Autodesk Inventor part; units mm, degrees
ref_plane "YZ Plane" through (0, 0, 0) normal (1, 0, 0) x (0, 1, 0)
ref_plane "XZ Plane" through (0, 0, 0) normal (0, 1, 0) x (-1, 0, 0)
ref_plane "XY Plane" through (0, 0, 0) normal (0, 0, 1) x (1, 0, 0)
sketch "Sketch1" plane through (0, 0, 0) normal (0, 1, 0) x (-1, 0, 0)
  line L0 (-21, 23) -> (21, 23)
  line L1 (21, 23) -> (21, -23)
  line L2 (21, -23) -> (-21, -23)
  line L3 (-21, -23) -> (-21, 23)
  line L4 (-21, 23) -> (21, -23) construction
  line L5 (21, 23) -> (-21, -23) construction
  point P0 (0, 0)
  dimension "d0" = 42
  dimension "d1" = 46
extrude "wall3" add sketch "Sketch1" along normal blind 4
fillet "Fillet6" radius 2 1 edges at (-21, 2, -23)
fillet "Fillet7" radius 2 1 edges at (21, 2, -23)
fillet "Fillet8" radius 2 1 edges at (-21, 2, 23)
fillet "Fillet9" radius 2 1 edges at (21, 2, 23)
sketch "Sketch10" plane through (0, 4, 0) normal (0, 1, 0) x (1, 0, 0)
  line L0 (-20.8799, 11) -> (21, 11) construction
  line L1 (21, -21) -> (21, 21)
  line L2 (14.0018, 23) -> (14.0018, -23) construction
  line L3 (-19, -23) -> (19, -23)
  line L4 (19, 23) -> (-19, 23)
  line L5 (-21, 19) -> (16, 19)
  line L6 (16, 19) -> (16, 3)
  line L7 (16, 3) -> (-21, 3)
  line L8 (-21, 3) -> (-21, 19)
  line L9 (-21, 19) -> (16, 3) construction
  line L10 (16, 19) -> (-21, 3) construction
  line L11 (-21, 21) -> (-21, -21)
  point P0 (0, 0)
  point P1 (-2.5, 11)
  dimension "d98" = 34
  dimension "d99" = 16
  dimension "d100" = 5
extrude "Extrusion8" cut sketch "Sketch10" against normal blind 2
sketch "Sketch12" plane through (-21, 0, -21) normal (-1, 0, 0) x (0, 0, 1)
  line L0 (17.9475, 1.9908) -> (19.9475, 1.9908)
  line L1 (19.9475, 1.9908) -> (19.9475, 3.0908)
  line L2 (19.9475, 3.0908) -> (17.9475, 3.0908)
  line L3 (17.9475, 3.0908) -> (17.9475, 1.9908)
  line L4 (2, 2) -> (0, 2)
  line L5 (0, 2) -> (0, 3.1)
  line L6 (0, 3.1) -> (2, 3.1)
  line L7 (2, 3.1) -> (2, 2)
  point P0 (21, 0)
  dimension "d102" = 0
  dimension "d103" = 2
  dimension "d104" = 1.1
  dimension "d105" = 2
  dimension "d106" = 1.1
extrude "Extrusion9" cut sketch "Sketch12" against normal blind 37
equation "\"d0\" = wallw"
equation "\"d72\" = wall3_thick"
equation "\"d89\" = cornerrad"
equation "\"d90\" = cornerrad"
equation "\"d91\" = cornerrad"
equation "\"d92\" = cornerrad"
equation "\"d98\" = distancefrombottom"
equation "\"d99\" = adapterh"
equation "\"d100\" = -0.5 * adapterw + 0.5 * wallw"
equation "\"d101\" = wall3slotd"
equation "\"d104\" = d106"
equation "\"printer3dtolerance\" = 0.1"
equation "\"wallw\" = 42"
equation "\"wallh\" = 44"
equation "\"cornerrad\" = 2"
equation "\"baseextra\" = 2"
equation "\"wall1_thick\" = 8"
equation "\"wall2_thick\" = 6.4"
equation "\"wall3_thick\" = 4"
equation "\"wall1slot\" = 8.1"
equation "\"wall2slot\" = 6.5"
equation "\"wall3slot\" = 4.1"
equation "\"gap2\" = 28"
equation "\"baseh\" = 79"
equation "\"basew\" = 44"
equation "\"base_thick\" = 6"
equation "\"base_slots_depth\" = 4"
equation "\"servomounth\" = 4"
equation "\"servosmallcircledia\" = 5.9"
equation "\"servomountsquare\" = 4"
equation "\"servobigcircledia\" = 11.6"
equation "\"servo9gw\" = 22.8"
equation "\"distancefromleft\" = 22"
equation "\"servopolygonl\" = 5.9"
equation "\"servopolygonr\" = 6.1"
equation "\"distancefrombottom\" = 34"
equation "\"d49\" = distancefrombottom"
equation "\"adapterh\" = 16"
equation "\"adapterw\" = 32"
equation "\"wall3slotw\" = 36"
equation "\"wall3slotd\" = 2"
equation "\"armslotd\" = 2"
equation "\"armthick\" = 3"
equation "\"armw\" = 34"
equation "\"fanhs\" = 9.6"
equation "\"fanhb\" = 11"
equation "\"adapterwallslotd\" = 2"
equation "\"adapterwallthick\" = 6"
equation "\"hornscrewholed\" = 2"
equation "\"armhornthick\" = 3"
equation "\"hornthick\" = 1.5"
equation "\"hornscrewheadd\" = 3"
properties part number "wall-end" material "Wood (Oak)"
Part model, mm, in its own coordinate system. A direction names the side the tool comes from. Give positions to 0.01 mm unless a question says otherwise; leave off trailing zeros. Write each loop counter-clockwise with the first axis right and the second up, starting at its lowest first coordinate (ties: lowest second). Pieces come first, ordered by that corner, then holes.
1) Probe L1, parallel to Z at x = -12, y = 2.05; L2, parallel to Z at x = -3, y = 3.55; L3, parallel to Y at x = 3.5, z = -5. List the from-to ranges inside material, lowest first.
Resolved:
L1: z = -23 to -21, -1.05 to 23
L2: z = -23 to -19, -3 to 23
L3: y = 0 to 2
2) Which spindle directions (+Z, -Z, +X, -X, +Y, -Y) get a long thin tool onto all of the face, cutting with end or side? Do faces 5 (the face through (-20.43, 2.03, 22.4)), 6 (the face through (-3, 3.091, -2)). Say none if no direction does.
Resolved:
face 5: +Z, -X, +Y, -Y
face 6: -X
3) Cut at B-B on z = -6. Write the cut outline in (x, y), then the cut area to 3 significant figures.
Resolved:
outline: (-21, 0) - (21, 0) - (21, 4) - (16, 4) - (16, 2) - (-21, 2) - close
area: 94.0 mm2
4) Two-plate mould, pull along Y, no slides. Class faces 1 (the face through (0, 4, 5)), 2 (the face through (-3, 1.991, -2)), 3 (the face through (-20.4, 2.03, -22.43)), 4 (the face through (-3, 3.1, -20)): released by +Y, released by -Y, zero draft, split by the parting line, or undercut.
Resolved:
face 1: released by +Y
face 2: undercut
face 3: zero draft
face 4: undercut
5) Pin check, flat tip, straight feed: pin 1 (1 mm diameter, centred on y = 3.5, z = -14, fed in from -X). Stop position of the tip, or through.
Resolved:
pin 1: stops at x = 16
